Input: part model. Units: mm. Frame: model coordinates. A direction names the side the tool comes from. Give positions to 0.01 mm unless a question says otherwise; leave off trailing zeros. Order: outer loops, then holes, each group sorted by start corner. A loop starts at its lowest first (then second) coordinate and runs counter-clockwise, first axis right, second up.
Autodesk Inventor part; units mm, degrees
ref_plane "YZ Plane" through (0, 0, 0) normal (1, 0, 0) x (0, 1, 0)
ref_plane "XZ Plane" through (0, 0, 0) normal (0, 1, 0) x (-1, 0, 0)
ref_plane "XY Plane" through (0, 0, 0) normal (0, 0, 1) x (1, 0, 0)
sketch "Sketch1" plane through (0, 0, 0) normal (1, 0, 0) x (0, 1, 0)
  circle A0 centre (0, 0) radius 3.5
  dimension "d7" = 7
extrude "Extrusion1" add sketch "Sketch1" along normal blind 10
sketch "Sketch2" plane through (0, 0, 0) normal (-1, 0, 0) x (0, 0, 1)
  line L0 (2.0913, 1.859) -> (-2.064, 1.859)
  line L1 (-2.064, 1.859) -> (-2.064, -1.6403)
  line L2 (-2.064, -1.6403) -> (2.0913, -1.6403)
  line L3 (2.0913, -1.6403) -> (2.0913, 1.859)
  point P0 (0, 0)
sketch "Sketch4" plane through (10, 0, 0) normal (1, 0, 0) x (0, 0, -1)
  point P0 (0, 0)
extrude "Extrusion2" cut sketch "Sketch2" against normal blind 16.25
properties part number "Wkp 01.03"
1) First-contact query: P1, Ø2, axis at x = 6, z = 2.5, coming from the -Y side; P2, Ø2, axis at x = 5, z = 1.5, coming from the +Y side. Flat tips, straight axial feed; report the tip coordinate or a pass-through.
2) Line query: probe 1 along Z at (x, y) = (5.75, 0); probe 2 along Z at (x, y) = (3, 1.25); probe 3 along Y at (x, z) = (7, 2). Output: solid intervals per line, ascending.
3) Cut plane B-B (y = 0). Return the cut outline in (x, z).
4) Pull-direction query (Z, two-part tool) for faces 1 (the face through (0, 0, -2.3)), 2 (the face through (4.93, 3.233, 1.341)), 3 (the face through (5, 0, 2.091)), 4 (the face through (5, 0, -2.064)); classes: pulls with the +Z half, pulls with the -Z half, needs draft (parallel to the pull), parting line crosses it, or undercut.
5) Cut plane D-D (y = -2.5). Return the cut outline in (x, z).
6) Cut plane C-C (x = 4). Return the cut outline in (y, z).
7) Reachability of faces 5 (the face through (5, 1.859, 0)), 6 (the face through (10, 0, -2.3)) from +Z, -Z, +X, -X, +Y, -Y: full face, straight path, thin tool, end or side. Return the list, or none.
8) Cut plane A-A (z = 0). Return the cut outline in (x, y).
Geometry says:
1. P1: stops at y = -3.16
1. P2: stops at y = 3.46
2. probe 1: z = -3.5 to -2.06, 2.09 to 3.5
2. probe 2: z = -3.27 to -2.06, 2.09 to 3.27
2. probe 3: y = -2.87 to -1.64, 1.86 to 2.87
3. outline: (0, -3.5) - (10, -3.5) - (10, -2.06) - (0, -2.06) - close; (0, 2.09) - (10, 2.09) - (10, 3.5) - (0, 3.5) - close
4. face 1: needs draft
4. face 2: parting line crosses it
4. face 3: undercut
4. face 4: undercut
5. outline: (0, -2.45) - (10, -2.45) - (10, 2.45) - (0, 2.45) - close
6. outline: circle Ø7 at (0, 0); hole (-1.64, -2.06) - (1.86, -2.06) - (1.86, 2.09) - (-1.64, 2.09) - close
7. face 5: +X, -X
7. face 6: +Z, -Z, +X, +Y, -Y
8. outline: (0, -3.5) - (10, -3.5) - (10, -1.64) - (0, -1.64) - close; (0, 1.86) - (10, 1.86) - (10, 3.5) - (0, 3.5) - close
